Can you work these out from the drawing? Everything is in mm from the part's minimum corner. Round coordinates to 2 decimals unless told otherwise and drop trailing zeros. Loops run counter-clockwise (first coordinate to the right, second up) from the corner with the lowest first, then second, coordinate; pieces in that order, holes last. Notation, with made-up numbers: M 70,-19 L 96,-19 A30 cw 96,19 Z; hole C -39.5,66 d6. An arc over 180 degrees is marked long. Use a Markdown table: item, result.
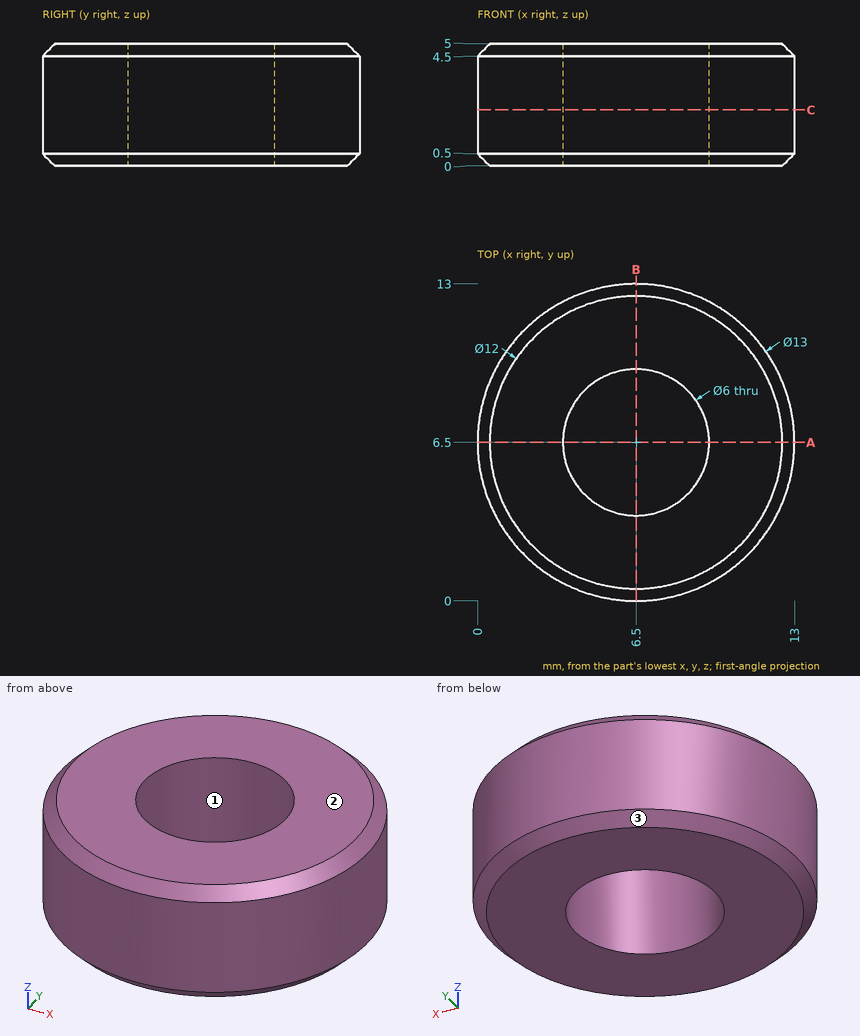
Q1. I need wall thicknesses on line 1 (Y direction, x = 6.5, z = 2.15); line 2 (X direction, y = 4.5, z = 2.85); line 3 (X direction, y = 4, z = 2.1). Which ranges of each line are inside material? Lowest first, please. Write a range as from..to.
Return value:
| item | result |
|---|---|
| line 1 | y = 0..3.5, 9.5..13 |
| line 2 | x = 0.32..4.26, 8.74..12.68 |
| line 3 | x = 0.5..4.84, 8.16..12.5 |
Q2. We'd pull the mould along Y, two halves only. Please class the marked faces 1, 2 and 3: pulls with the +Y half, pulls with the -Y half, needs draft (parallel to the pull), parting line crosses it, or undercut.
Return value:
| item | result |
|---|---|
| face 1 | undercut |
| face 2 | needs draft |
| face 3 | parting line crosses it |
Q3. Imagine slicing it at C-C, the plane z = 2.3. Please give me the cut outline in (x, y).
Return value:
| item | result |
|---|---|
| outline | C 6.5,6.5 d13; hole C 6.5,6.5 d6 |
Q4. Will this pin go through, and if not, where does the flat tip stop? P1, Ø1.5, axis at x = 10.5, z = 2.5, coming from the -Y side.
Return value:
| item | result |
|---|---|
| P1 | stops at y = 0.87 |
Q5. Imagine slicing it at A-A, the plane y = 6.5. Please give me the cut outline in (x, z), then the cut area to 3 significant figures.
Return value:
| item | result |
|---|---|
| outline | M 0,0.5 L 0.5,0 L 3.5,0 L 3.5,5 L 0.5,5 L 0,4.5 Z; M 9.5,0 L 12.5,0 L 13,0.5 L 13,4.5 L 12.5,5 L 9.5,5 Z |
| area | 34.5 mm^2 |
